Could you check a few things on this model? Use its own coordinates, in mm. Round coordinates to 2 decimals unless told otherwise and drop trailing zeros. Write each loop counter-clockwise with the first axis right and the second up, starting at its lowest first coordinate (ties: lowest second). Pieces come first, ordered by that corner, then holes. Notation, with made-up numbers: M 6.25,74.25 L 58.25,74.25 A17 cw 58.25,103.25 Z; hole C 77.5,-21 d9. An arc over 180 degrees is marked long. One line per item, written item: value. Start each with the question number.
(1) I'm going to push flat-ended pins straight in: pin 1 Ø0.9 at (y, z) = (1.5, -5.5) entering from +X; pin 2 Ø1.5 at (x, y) = (-2.5, 1) entering from -Z; pin 3 Ø0.9 at (x, y) = (18, 1) entering from -Z. Where does each tip first touch, or does it pass through?
(2) If I drill on L1, parallel to X at y = 1, z = 21; L2, parallel to X at y = 0.4, z = 7.5; L3, parallel to Z at x = -19.5, y = 1.6, over which ranges is the centre line in solid material (lowest first)?
(3) I want a section at B-B on z = 14.5. Please give me the cut outline in (x, y).
(4) I want a section at D-D on x = 14. Please give me the cut outline in (y, z), and give its area (3 significant figures).
(5) I want a section at C-C on x = -7. Please give me the cut outline in (y, z), and give its area (3 significant figures).
(6) I want a section at A-A on z = 0. Please give me the cut outline in (x, y), and give its area (3 significant figures).
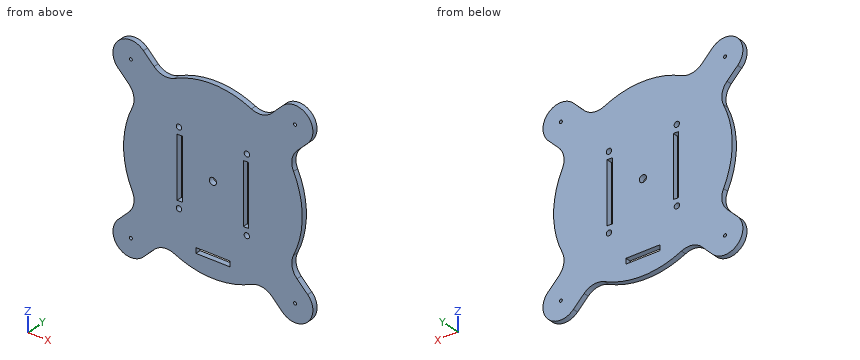
```python
from build123d import *

# Parameters (mm, degrees)
ESQUISSE1_R        = 0.85
ESQUISSE1_R_2      = 1.5
ESQUISSE1_R_3      = 2
ESQUISSE1_W        = 3
ESQUISSE1_H        = 34
ESQUISSE1_W_2      = 19
ESQUISSE1_H_2      = 3
BOSS_EXTRU_1_DEPTH = 3
CONG_1_R           = 10


with BuildPart() as part:
    # Esquisse1 → Boss.-Extru.1 (new body)
    with BuildSketch(Plane(origin=(0, 0, 0), x_dir=(1, 0, 0), z_dir=(0, 1, 0))):
        with BuildLine():
            Line((-38.890872965, -53.033008589), (-27.56994834, -41.712083963))
            ThreePointArc((-27.56994834, -41.712083963), (0, -50), (27.56994834, -41.712083963))
            Line((27.56994834, -41.712083963), (38.890872965, -53.033008589))
            ThreePointArc((38.890872965, -53.033008589), (53.033008589, -53.033008589), (53.033008589, -38.890872965))
            Line((53.033008589, -38.890872965), (41.712083963, -27.56994834))
            ThreePointArc((41.712083963, -27.56994834), (50, 0), (41.712083963, 27.56994834))
            Line((41.712083963, 27.56994834), (53.033008589, 38.890872965))
            ThreePointArc((53.033008589, 38.890872965), (53.033008589, 53.033008589), (38.890872965, 53.033008589))
            Line((38.890872965, 53.033008589), (27.56994834, 41.712083963))
            ThreePointArc((27.56994834, 41.712083963), (0, 50), (-27.56994834, 41.712083963))
            Line((-27.56994834, 41.712083963), (-38.890872965, 53.033008589))
            ThreePointArc((-38.890872965, 53.033008589), (-53.033008589, 53.033008589), (-53.033008589, 38.890872965))
            Line((-53.033008589, 38.890872965), (-41.712083963, 27.56994834))
            ThreePointArc((-41.712083963, 27.56994834), (-50, 0), (-41.712083963, -27.56994834))
            Line((-41.712083963, -27.56994834), (-53.033008589, -38.890872965))
            ThreePointArc((-53.033008589, -38.890872965), (-53.033008589, -53.033008589), (-38.890872965, -53.033008589))
        make_face()
        with Locations(Location((-45.961940777, -45.961940777, 0), (0, 0, 270))):
            Circle(ESQUISSE1_R, mode=Mode.SUBTRACT)
        with Locations(Location((-45.961940777, 45.961940777, 0), (0, 0, 270))):
            Circle(ESQUISSE1_R, mode=Mode.SUBTRACT)
        with Locations(Location((45.961940777, 45.961940777, 0), (0, 0, 270))):
            Circle(ESQUISSE1_R, mode=Mode.SUBTRACT)
        with Locations(Location((45.961940777, -45.961940777, 0), (0, 0, 270))):
            Circle(ESQUISSE1_R, mode=Mode.SUBTRACT)
        with Locations(Location((-19, 21, 0), (0, 0, 270))):
            Circle(ESQUISSE1_R_2, mode=Mode.SUBTRACT)
        with Locations(Location((19, 21, 0), (0, 0, 270))):
            Circle(ESQUISSE1_R_2, mode=Mode.SUBTRACT)
        with Locations(Location((19, -21, 0), (0, 0, 270))):
            Circle(ESQUISSE1_R_2, mode=Mode.SUBTRACT)
        with Locations(Location((-19, -21, 0), (0, 0, 270))):
            Circle(ESQUISSE1_R_2, mode=Mode.SUBTRACT)
        with Locations(Location((0, 0, 0), (0, 0, 270))):
            Circle(ESQUISSE1_R_3, mode=Mode.SUBTRACT)
        with Locations((-18.5, 0)):
            Rectangle(ESQUISSE1_W, ESQUISSE1_H, mode=Mode.SUBTRACT)
        with Locations((18.5, 0)):
            Rectangle(ESQUISSE1_W, ESQUISSE1_H, mode=Mode.SUBTRACT)
        with Locations((0, 39)):
            Rectangle(ESQUISSE1_W_2, ESQUISSE1_H_2, mode=Mode.SUBTRACT)
    extrude(amount=BOSS_EXTRU_1_DEPTH)

    # Congé1
    cong_1_edges = [part.edges().sort_by_distance(p)[0] for p in [
        (-27.56994834, 1.5, 41.712083963),
        (-41.712083963, 1.5, 27.56994834),
        (-41.712083963, 1.5, -27.56994834),
        (-27.56994834, 1.5, -41.712083963),
        (27.56994834, 1.5, -41.712083963),
        (41.712083963, 1.5, -27.56994834),
        (41.712083963, 1.5, 27.56994834),
        (27.56994834, 1.5, 41.712083963),
    ]]
    fillet(cong_1_edges, radius=CONG_1_R)


solid = part.part
```
Found:
1. pin 1: stops at x = 49.74
1. pin 2: stops at z = -49.97
1. pin 3: stops at z = -46.82
2. L1: x = -45.38 to -20.5, -17.5 to 17.5, 20.5 to 45.38
2. L2: x = -49.43 to -20, -17 to 17, 20 to 49.43
2. L3: z = -46.04 to -22.41, -19.59 to -17, 17 to 19.59, 22.41 to 46.04
3. outline: M -47.85,0 L -20,0 L -20,3 L -47.85,3 Z; M -17,0 L 17,0 L 17,3 L -17,3 Z; M 20,0 L 47.85,0 L 47.85,3 L 20,3 Z
4. outline: M 0,-48 L 3,-48 L 3,48 L 0,48 Z
4. area: 288 mm²
5. outline: M 0,-49.51 L 3,-49.51 L 3,-40.5 L 0,-40.5 Z; M 0,-37.5 L 3,-37.5 L 3,49.51 L 0,49.51 Z
5. area: 288 mm²
6. outline: M -50,0 L -20,0 L -20,3 L -50,3 Z; M -17,0 L -2,0 L -2,3 L -17,3 Z; M 2,0 L 17,0 L 17,3 L 2,3 Z; M 20,0 L 50,0 L 50,3 L 20,3 Z
6. area: 270 mm²
